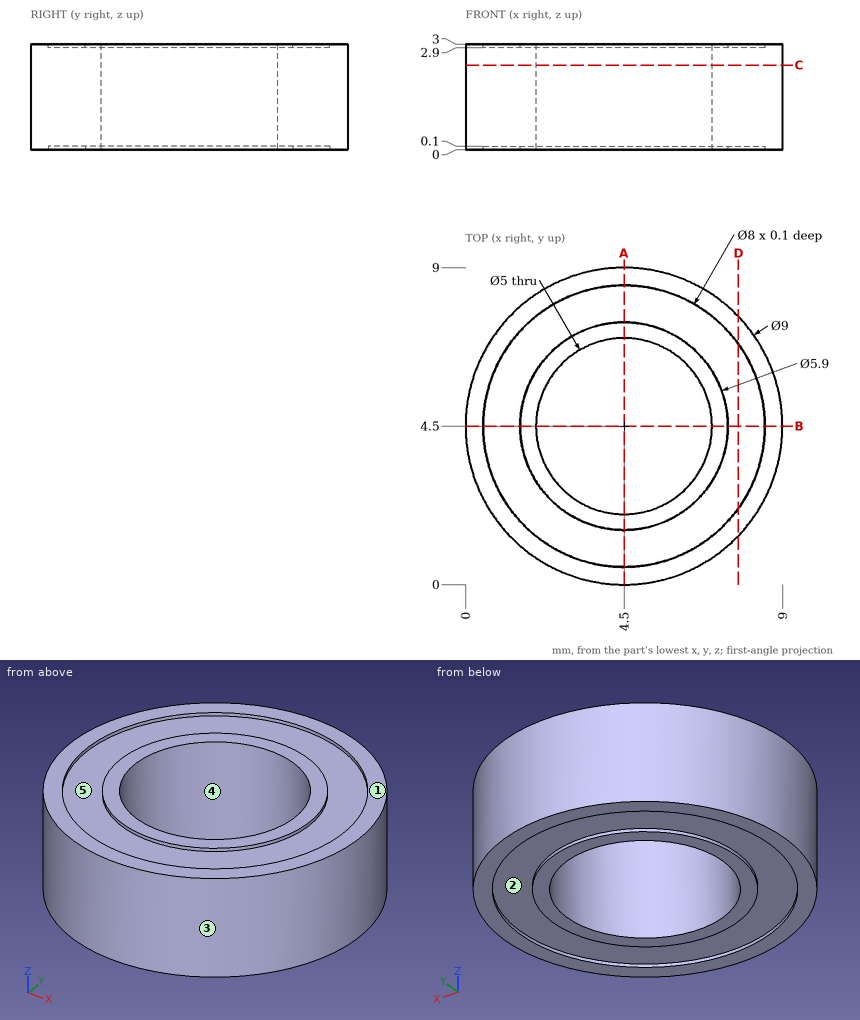
Study the drawing (mm; zero at the part's minimum x, y, z) and answer. A direction names the side the tool comes from. Give positions to 0.01 mm unless a question says otherwise; leave off trailing zeros. Write each loop counter-clockwise with the first axis right and the second up, starting at its lowest first coordinate (ties: lowest second). Pieces come first, ordered by that corner, then holes.
Item 1: Section A-A, the plane x = 4.5 is taken. Write down the section's boundary in (y, z).
Item 2: Find the intervals of material crossed by line 1 along Y through (x, z) = (4.5, 1.1); line 2 along Z through (x, y) = (8.25, 4); line 3 along X through (y, z) = (2.5, 2.7), in increasing order.
Item 3: Section D-D, the plane x = 7.75 is taken. Write down the section's boundary in (y, z), plus the area to 3 significant figures.
Item 4: Which of the six approach directions +Z, -Z, +X, -X, +Y, -Y give full straight-line access (tool end or side, diameter ignored) to the marked faces 4 and 5?
Item 5: Determine the mould class of the marked faces 1, 2 and 3 for opening direction X: released by +X, released by -X, zero draft, split by the parting line, or undercut.
Item 6: Section C-C, the plane z = 2.4 is taken. Write down the section's boundary in (x, y).
Item 7: Flat-ended cylindrical pins translate along their axes: P1, Ø4, axis at x = 5.5, y = 6, coming from the -Z side; P2, Ø1, axis at y = 5.5, z = 1.5, coming from the +X side. Find the tip coordinate at first contact, or state that the pin passes through.
Completed:
1. outline: (0, 0) - (0.5, 0) - (0.5, 0.1) - (1.55, 0.1) - (1.55, 0) - (2, 0) - (2, 3) - (1.55, 3) - (1.55, 2.9) - (0.5, 2.9) - (0.5, 3) - (0, 3) - close; (7, 0) - (7.45, 0) - (7.45, 0.1) - (8.5, 0.1) - (8.5, 0) - (9, 0) - (9, 3) - (8.5, 3) - (8.5, 2.9) - (7.45, 2.9) - (7.45, 3) - (7, 3) - close
2. line 1: y = 0 to 2, 7 to 9
2. line 2: z = 0.1 to 2.9
2. line 3: x = 0.47 to 3, 6 to 8.53
3. outline: (1.39, 0) - (2.17, 0) - (2.17, 0.1) - (6.83, 0.1) - (6.83, 0) - (7.61, 0) - (7.61, 3) - (6.83, 3) - (6.83, 2.9) - (2.17, 2.9) - (2.17, 3) - (1.39, 3) - close
3. area: 17.7 mm2
4. face 4: +Z, -Z
4. face 5: +Z
5. face 1: zero draft
5. face 2: undercut
5. face 3: split by the parting line
6. outline: circle Ø9 at (4.5, 4.5); hole circle Ø5 at (4.5, 4.5)
7. P1: stops at z = 0
7. P2: stops at x = 8.97
